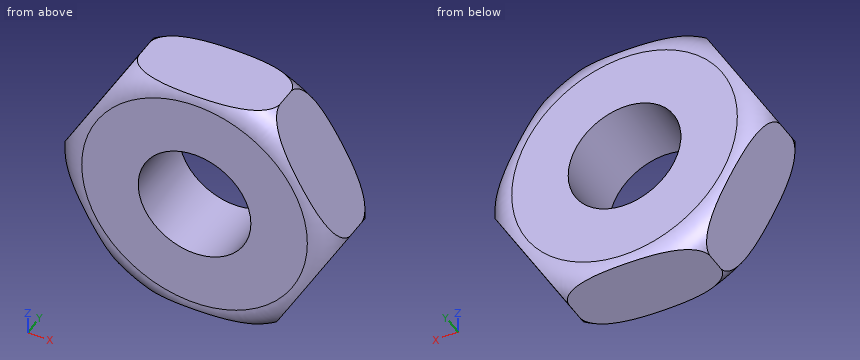
from build123d import *

# Parameters (mm, degrees)
SKETCH1_R           = 6
BOSS_EXTRUDE1_DEPTH = 4


with BuildPart() as part:
    # Sketch1 → Boss-Extrude1 (new body, symmetric)
    with BuildSketch(Plane(origin=(0, 0, 0), x_dir=(1, 0, 0), z_dir=(0, 1, 0))):
        Polygon((15.011106999, 0), (7.505553499, 13), (-7.505553499, 13), (-15.011106999, 0), (-7.505553499, -13), (7.505553499, -13), align=None)
        Circle(SKETCH1_R, mode=Mode.SUBTRACT)
    extrude(amount=BOSS_EXTRUDE1_DEPTH, both=True)

    # Sketch2 → Cut-Revolve1 (revolve, cut)
    with BuildSketch(Plane.XY):
        with BuildLine():
            Line((15.011106999, 4), (15.011106999, 1))
            ThreePointArc((15.011106999, 1), (14.132427342, 3.121320344), (12.011106999, 4))
            Line((12.011106999, 4), (15.011106999, 4))
        make_face()
    cut_revolve1 = revolve(axis=Axis((0, 0, 0), (0, -1, 0)), mode=Mode.SUBTRACT)

    # Mirror1: Cut-Revolve1 across plane
    add(cut_revolve1.mirror(Plane.ZX), mode=Mode.SUBTRACT)


solid = part.part
Here's how the part is built. I have some questions about the finished solid (model axes, mm). Coordinates: 2 decimals unless noted, no trailing zeros. Write each loop counter-clockwise with the first axis right and the second up, starting at its lowest first coordinate (ties: lowest second). Pieces come first, ordered by that corner, then holes.
Item 1: Will these pins go through, and if not, where does the flat tip stop? pin 1 (4 mm diameter, centred on x = -11.5, z = -9, fed in from -Y); pin 2 (4 mm diameter, centred on x = -9, y = 3, fed in from +Z).
Item 2: If I drill on line 1 (Z direction, x = 0, y = -0.25); line 2 (X direction, y = -1.5, z = 0); line 3 (X direction, y = 2.75, z = -1), over which ranges is the centre line in solid material (lowest first)?
Item 3: I want a section at C-C on y = -3.5. Write out the boundary of the cut face in (x, z).
Item 4: I want a section at A-A on x = 0. Write out the boundary of the cut face in (y, z).
Item 5: I want a section at B-B on y = -0.25. Write out the boundary of the cut face in (x, z).
Findings below:
1. pin 1: stops at y = -3.94
1. pin 2: stops at z = 12.94
2. line 1: z = -13 to -6, 6 to 13
2. line 2: x = -14.97 to -6, 6 to 14.97
2. line 3: x = -14.41 to -5.92, 5.92 to 14.41
3. outline: (-13.37, -2.84) - (-9.15, -10.16) arc R13.67 ccw to (-4.23, -13) - (4.23, -13) arc R13.67 ccw to (9.15, -10.16) - (13.37, -2.84) arc R13.67 ccw to (13.37, 2.84) - (9.15, 10.16) arc R13.67 ccw to (4.23, 13) - (-4.23, 13) arc R13.67 ccw to (-9.15, 10.16) - (-13.37, 2.84) arc R13.67 ccw to start; hole circle Ø12 at (0, 0)
4. outline: (-4, -12.01) arc R3 ccw to (-3.83, -13) - (3.83, -13) arc R3 ccw to (4, -12.01) - (4, -6) - (-4, -6) - close; (-4, 6) - (4, 6) - (4, 12.01) arc R3 ccw to (3.83, 13) - (-3.83, 13) arc R3 ccw to (-4, 12.01) - close
5. outline: (-15.01, 0) - (-7.51, -13) - (7.51, -13) - (15.01, 0) - (7.51, 13) - (-7.51, 13) - close; hole circle Ø12 at (0, 0)
